Here's how the part is built. I have some questions about the finished solid (model axes, mm). Coordinates: 2 decimals unless noted, no trailing zeros. Answer in a Markdown table with one row per item. Add a question column.
Item 1: Will these pins go through, and if not, where does the flat tip stop? pin 1 Ø3 at (x, y) = (7, 0) entering from -Z; pin 2 Ø3 at (y, z) = (3, 10) entering from -X; pin 3 Ø2 at (x, y) = (-7, 0) entering from +Z; pin 4 Ø1.5 at (x, z) = (-25.5, 6.5) entering from -Y.
Item 2: If I drill on line 1 along Y through (x, z) = (0, 7); line 2 along Y through (x, z) = (-16, 5.5); line 3 along Y through (x, z) = (7, 6.5), over which ranges is the centre line in solid material (lowest first)? Write a range as from..to.
Item 3: I want a section at A-A (z = 13). Count the separate pieces of the cut face and the enclosed holes in it, plus the area to 3 significant figures.
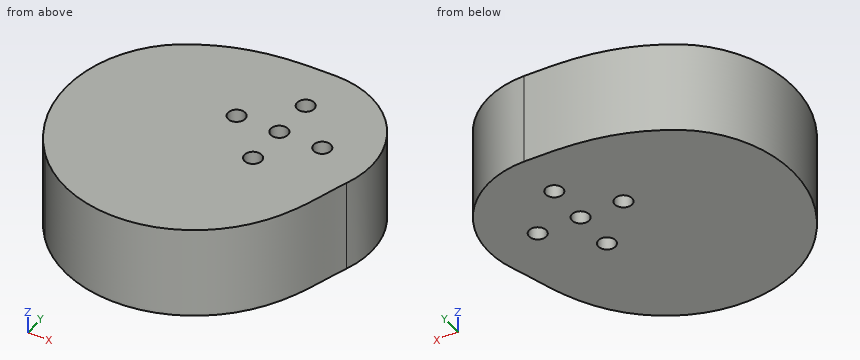
```python
from build123d import *

# Parameters (mm, degrees)
EXTRUDE_1_DEPTH     = 15
SKETCH_3_R          = 1.4
CUT_EXTRUDE_2_DEPTH = 45.491091955


with BuildPart() as part:
    # 草图1 → 凸台-拉伸1 (new body)
    with BuildSketch(Plane.XY):
        with BuildLine():
            ThreePointArc((14.095389312, -5.13030215), (12.287280664, 8.603646545), (0, 15))
            add(Edge.make_bspline(
                [(0, 15), (-0.174596768, 14.999999319), (-0.436611581, 14.999693042), (-0.786186323, 14.998643785), (-1.048915847, 14.997519085), (-1.312216235, 14.99603471), (-1.576228693, 14.994161918), (-1.84109342, 14.991865662), (-2.106949414, 14.989104591), (-2.373934268, 14.985831089), (-2.642183971, 14.981991319), (-2.911832716, 14.977525266), (-3.1830127, 14.972366794), (-3.455853932, 14.966443701), (-3.730484039, 14.959677782), (-4.007028071, 14.9519849), (-4.285608318, 14.943275054), (-4.566344116, 14.933452466), (-4.849351664, 14.922415656), (-5.134743838, 14.910057537), (-5.422630012, 14.896265505), (-5.713115875, 14.880921543), (-6.006303259, 14.863902316), (-6.302289959, 14.84507929), (-6.601169567, 14.824318836), (-6.903031299, 14.801482354), (-7.207959833, 14.776426392), (-7.516035146, 14.749002775), (-7.827332351, 14.719058736), (-8.141921549, 14.686437053), (-8.459867669, 14.650976187), (-8.781230323, 14.612510428), (-9.106063662, 14.570870045), (-9.434416233, 14.525881438), (-9.766330843, 14.477367292), (-10.101844426, 14.425146744), (-10.440987913, 14.36903554), (-10.783786108, 14.30884621), (-11.130257567, 14.244388236), (-11.480414483, 14.175468229), (-11.834262574, 14.101890107), (-12.191800976, 14.023455277), (-12.553022141, 13.939962822), (-12.917911738, 13.851209688), (-13.286448564, 13.756990875), (-13.658604451, 13.657099633), (-14.03434419, 13.551327657), (-14.413625446, 13.439465288), (-14.796398691, 13.321301714), (-15.182607133, 13.196625177), (-15.572186657, 13.065223175), (-15.965065767, 12.926882676), (-16.361165533, 12.781390325), (-16.760399548, 12.62853266), (-17.162673883, 12.468096321), (-17.567887059, 12.299868276), (-17.975930009, 12.12363602), (-18.386686074, 11.939187837), (-18.800030904, 11.746312879), (-19.21583277, 11.544801919), (-19.63395132, 11.334445536), (-20.054242271, 11.115042096), (-20.476539575, 10.886368472), (-20.900723293, 10.648292485), (-21.326461435, 10.400346233), (-21.753514654, 10.143757392), (-22.178049863, 9.87535726), (-22.595959424, 9.592299141), (-23.006858872, 9.296248411), (-23.410215858, 8.987163154), (-23.805723663, 8.665361009), (-24.19302422, 8.331073979), (-24.571782966, 7.984568061), (-24.94166894, 7.626110759), (-25.302360391, 7.255979562), (-25.65354351, 6.874459377), (-25.994913004, 6.481842935), (-26.326172169, 6.078430394), (-26.647033089, 5.664529144), (-26.957216795, 5.240453567), (-27.256453426, 4.80652479), (-27.544482381, 4.363070443), (-27.82105247, 3.910424411), (-28.085922052, 3.448926584), (-28.338859169, 2.978922599), (-28.579641679, 2.500763586), (-28.808057373, 2.014805906), (-29.023904095, 1.521410888), (-29.226989847, 1.020944566), (-29.417132895, 0.513777409), (-29.594161862, 0.000284053), (-29.757915818, -0.519156969), (-29.908244365, -1.044163505), (-30.045007708, -1.574350056), (-30.168076728, -2.109328051), (-30.277333041, -2.648706129), (-30.372669056, -3.192090415), (-30.453988019, -3.739084801), (-30.521204062, -4.289291227), (-30.574242228, -4.842309963), (-30.613038507, -5.39773989), (-30.637539851, -5.955178784), (-30.647704191, -6.514223598), (-30.643500444, -7.074470745), (-30.624908509, -7.63551638), (-30.591919266, -8.196956684), (-30.544534557, -8.758388145), (-30.48276717, -9.319407838), (-30.406640805, -9.879613709), (-30.316190047, -10.438604851), (-30.21146032, -10.995981785), (-30.092507839, -11.551346736), (-29.95939956, -12.104303912), (-29.812213112, -12.654459772), (-29.651036733, -13.201423307), (-29.475969194, -13.744806302), (-29.287119719, -14.284223615), (-29.084607895, -14.819293432), (-28.868563581, -15.349637541), (-28.639126801, -15.874881588), (-28.396447646, -16.394655341), (-28.140686152, -16.908592941), (-27.872012186, -17.416333158), (-27.590605319, -17.917519643), (-27.296654692, -18.411801174), (-26.990358881, -18.898831896), (-26.671925755, -19.378271573), (-26.341572303, -19.849785794), (-25.885480421, -20.467504768), (-25.526267712, -20.917866263), (-25.279466623, -21.21199112)],
                knots=[0, 0, 0, 0, 0.008983592, 0.013481544, 0.017986876, 0.022502032, 0.027029448, 0.031571543, 0.036130722, 0.040709366, 0.045309838, 0.049934477, 0.054585593, 0.059265472, 0.063976367, 0.068720504, 0.073500073, 0.078317234, 0.083174111, 0.088072793, 0.093015336, 0.098003759, 0.103040044, 0.108126138, 0.113263955, 0.118455369, 0.123702222, 0.129006319, 0.134369433, 0.139793302, 0.145279632, 0.150830096, 0.156446337, 0.162129965, 0.167882565, 0.173705688, 0.179600863, 0.185569587, 0.191613334, 0.197733555, 0.203931674, 0.210209093, 0.216567194, 0.223007337, 0.229530862, 0.236139089, 0.242833322, 0.249614847, 0.256484933, 0.263444834, 0.270495789, 0.277639024, 0.284875752, 0.292207171, 0.299634469, 0.307158825, 0.314781404, 0.322503362, 0.330325849, 0.338250002, 0.346276954, 0.354407827, 0.362643738, 0.370985797, 0.379435108, 0.387992769, 0.396619209, 0.405274739, 0.413959558, 0.422673829, 0.431417677, 0.440191194, 0.448994436, 0.457827427, 0.466690157, 0.475582587, 0.484504647, 0.493456237, 0.50243723, 0.511447469, 0.520486775, 0.529554938, 0.538651727, 0.547776885, 0.556930133, 0.566111169, 0.575319669, 0.584555288, 0.593817663, 0.603106409, 0.612421123, 0.621761385, 0.631126755, 0.64051678, 0.649930987, 0.659368891, 0.66882999, 0.678313767, 0.687819694, 0.697347228, 0.706895812, 0.71646488, 0.726053851, 0.735662137, 0.745289135, 0.754934234, 0.764596814, 0.774276244, 0.783971886, 0.793683092, 0.803409207, 0.813149569, 0.822903507, 0.832670344, 0.8424494, 0.852239983, 0.862041401, 0.871852953, 0.881673937, 0.891503642, 0.901341356, 0.911186363, 0.921037943, 0.930895373, 0.940757928, 0.95062488, 0.960495499, 0.970369054, 0.980244811, 1, 1, 1, 1], degree=3))
            add(Edge.make_bspline(
                [(-25.279466623, -21.21199112), (-25.03266702, -21.506118015), (-24.650058643, -21.936850324), (-24.116326131, -22.48889957), (-23.704647777, -22.89139552), (-23.281933222, -23.282038607), (-22.848561661, -23.660506241), (-22.404923763, -24.026490317), (-21.951421131, -24.379697722), (-21.48846567, -24.719850743), (-21.016478952, -25.046687464), (-20.535891561, -25.359962134), (-20.047142425, -25.659445508), (-19.550678137, -25.944925156), (-19.04695226, -26.216205747), (-18.536424623, -26.4731093), (-18.019560603, -26.715475403), (-17.496830406, -26.943161412), (-16.968708336, -27.156042604), (-16.435672059, -27.354012309), (-15.898201862, -27.536982008), (-15.35677991, -27.704881402), (-14.811889501, -27.857658441), (-14.264014323, -27.995279333), (-13.713637708, -28.117728512), (-13.161241887, -28.225008578), (-12.607307258, -28.317140209), (-12.052311649, -28.394162034), (-11.496729594, -28.456130483), (-10.941031611, -28.5031196), (-10.385683496, -28.535220833), (-9.831145623, -28.552542784), (-9.277872252, -28.555210939), (-8.726310862, -28.543367367), (-8.176901485, -28.517170386), (-7.630076062, -28.476794208), (-7.086257816, -28.422428554), (-6.545860639, -28.354278239), (-6.009288499, -28.272562744), (-5.476934872, -28.177515748), (-4.949182183, -28.069384646), (-4.426401286, -27.948430045), (-3.908950946, -27.814925234), (-3.397177365, -27.669155633), (-2.891413716, -27.511418228), (-2.391979716, -27.342020982), (-1.899181211, -27.161282232), (-1.413309805, -26.969530066), (-0.934642496, -26.767101692), (-0.463441361, -26.554342786), (4.6748e-05, -26.331606829), (0.455590466, -26.099254437), (0.902974156, -25.857652676), (1.341998114, -25.607174371), (1.77247875, -25.348197408), (2.194248731, -25.081104026), (2.607157097, -24.806280109), (3.011069352, -24.524114474), (3.405867507, -24.234998154), (3.791450116, -23.939323681), (4.167732256, -23.637484373), (4.534645494, -23.329873622), (4.892137816, -23.016884179), (5.240173528, -22.698907455), (5.578733117, -22.376332816), (5.907813101, -22.049546899), (6.22742583, -21.71893292), (6.537599266, -21.384870008), (6.838376738, -21.047732541), (7.129816662, -20.707889495), (7.411992235, -20.365703811), (7.684991105, -20.021531772), (7.948915008, -19.675722401), (8.20387939, -19.32861687), (8.450012994, -18.980547932), (8.687457427, -18.631839373), (8.916366703, -18.282805481), (9.136906768, -17.933750534), (9.349254998, -17.58496832), (9.553599678, -17.236741672), (9.750139466, -16.889342026), (9.939082834, -16.543029011), (10.120647493, -16.198050057), (10.295059808, -15.854640037), (10.462554187, -15.513020927), (10.623372469, -15.173401503), (10.777763289, -14.835977057), (10.925981441, -14.50092915), (11.068287227, -14.168425389), (11.204945795, -13.838619231), (11.336226478, -13.511649827), (11.462402118, -13.187641886), (11.583748391, -12.866705573), (11.70054313, -12.548936438), (11.813065642, -12.234415378), (11.921596028, -11.923208621), (12.026414502, -11.615367753), (12.127800711, -11.310929767), (12.226033064, -11.009917143), (12.321388061, -10.712337965), (12.414139626, -10.418186058), (12.504558455, -10.127441167), (12.592911364, -9.840069152), (12.679460654, -9.556022225), (12.76446348, -9.275239204), (12.848171238, -8.997645806), (12.93082896, -8.723154954), (13.01267473, -8.451667126), (13.093939106, -8.183070715), (13.174844564, -7.917242422), (13.255604965, -7.654047671), (13.336425025, -7.393341046), (13.417499824, -7.134966749), (13.49901432, -6.87875908), (13.581142893, -6.624542932), (13.664048917, -6.372134315), (13.747884322, -6.121340875), (13.832789331, -5.871962488), (13.947500586, -5.541332702), (14.035654827, -5.294414261), (14.095389312, -5.13030215)],
                knots=[0, 0, 0, 0, 0.021270399, 0.031903677, 0.042534645, 0.053162531, 0.063786554, 0.074405932, 0.085019874, 0.095627584, 0.106228257, 0.116821079, 0.127405228, 0.137979868, 0.148544155, 0.15909723, 0.169638222, 0.180166248, 0.190680407, 0.201179787, 0.211663457, 0.222130473, 0.232579872, 0.243010676, 0.253421887, 0.263812492, 0.27418146, 0.284527741, 0.294850266, 0.30514795, 0.315419689, 0.32566436, 0.335880824, 0.346067921, 0.356224476, 0.366349296, 0.376441173, 0.386498878, 0.396521172, 0.406506796, 0.416454478, 0.426362934, 0.436230863, 0.446056956, 0.45583989, 0.465578331, 0.475270938, 0.48491636, 0.49451324, 0.504060215, 0.513555916, 0.522998973, 0.532388013, 0.541721663, 0.550998551, 0.560217309, 0.569376572, 0.578474983, 0.587511192, 0.596483859, 0.605391658, 0.614233274, 0.623007411, 0.631712789, 0.640348151, 0.64891226, 0.657403907, 0.66582191, 0.674165115, 0.682432404, 0.690622694, 0.69873494, 0.706768137, 0.714721328, 0.7225936, 0.730384093, 0.738092, 0.745716573, 0.753257123, 0.760713027, 0.76808373, 0.775368751, 0.782567685, 0.789680206, 0.796706075, 0.803645143, 0.810497353, 0.81726275, 0.823941479, 0.830533798, 0.837040075, 0.8434608, 0.849796585, 0.856048172, 0.86221644, 0.868302406, 0.874307234, 0.880232236, 0.886078882, 0.891848803, 0.897543794, 0.903165817, 0.908717009, 0.914199683, 0.919616328, 0.924969613, 0.930262387, 0.935497677, 0.94067869, 0.945808804, 0.950891568, 0.955930696, 0.960930056, 0.965893662, 0.970825666, 0.975730339, 0.980612064, 0.985475315, 0.990324642, 1, 1, 1, 1], degree=3))
        make_face()
    extrude(amount=EXTRUDE_1_DEPTH)

    # 草图3 → 切除-拉伸2 (cut, through all)
    with BuildSketch(Plane.XY.offset(15)):
        Circle(SKETCH_3_R)
        with Locations((7, 0)):
            Circle(SKETCH_3_R)
        with Locations((0, -7)):
            Circle(SKETCH_3_R)
        with Locations((-7, 0)):
            Circle(SKETCH_3_R)
        with Locations((0, 7)):
            Circle(SKETCH_3_R)
    extrude(amount=-CUT_EXTRUDE_2_DEPTH, mode=Mode.SUBTRACT)


solid = part.part
```
Values follow:
| question | item | result |
|---|---|---|
| 1 | pin 1 | stops at z = 0 |
| 1 | pin 2 | stops at x = -29.03 |
| 1 | pin 3 | passes through |
| 1 | pin 4 | stops at y = -21.82 |
| 2 | line 1 | y = -26.33..-8.4, -5.6..-1.4, 1.4..5.6, 8.4..15 |
| 2 | line 2 | y = -27.5..12.91 |
| 2 | line 3 | y = -20.86..-1.4, 1.4..13.27 |
| 3 | separate pieces | 1 |
| 3 | enclosed holes | 5 |
| 3 | area | 1,530 mm^2 |
